Verification items for the finished model (mm, model axes). Coordinates: 2 decimals unless noted, no trailing zeros. Order: outer loops, then holes, each group sorted by start corner. A loop starts at its lowest first (then second) coordinate and runs counter-clockwise, first axis right, second up.
Q1. Cross-section at B-B, the plane x = 5. Record the boundary of the cut face in (y, z).
Q2. Cross-section at C-C, the plane y = 0.75. Record the boundary of the cut face in (x, z).
Q3. Thickness scan on line 1 (X direction, y = 2.65, z = 3); line 2 (Z direction, x = 17, y = 1.95). Record the ranges inside material, lowest first.
Q4. Depth check by flat-ended pin: P1, Ø2.5, axis at x = 17, z = 11, coming from the +Y side. Enter the tip coordinate at first touch or a pass-through.
Q5. Cross-section at A-A, the plane z = 3. Record the boundary of the cut face in (x, y).
Q6. Draft check along Z on faces 1 (the cylindrical face through (15.5, 1.97, 3.07)), 2 (the cylindrical face through (15.5, 1.97, 11.07)), 3 (the flat face through (11, 4, 7)), 4 (the flat face through (11, 2, 0)). Enter one of: pulls with the +Z half, pulls with the -Z half, needs draft (parallel to the pull), parting line crosses it, or undercut.
Autodesk Fusion 360 part; units mm, degrees
sketch "Sketch1" plane through (0, 0, 0) normal (0, 1, 0) x (1, 0, 0)
  line L0 (0, 0) -> (22, 0)
  line L1 (22, 0) -> (22, -15)
  line L2 (22, -15) -> (0, -15)
  line L3 (0, -15) -> (0, 0)
  circle A0 centre (17, -11) radius 1.5
  line L4 (0, -15) -> (0, -14.748)
  circle A1 centre (5, -3) radius 1.5
  circle A2 centre (17, -3) radius 1.5
  circle A3 centre (5, -11) radius 1.5
  dimension "d11" = 3
  dimension "d18" = 3
  dimension "d21" = 3
  dimension "d24" = 3
extrude "Extrude1" add sketch "Sketch1" along normal blind 4 makes body 1
copy_body "Body->Comp1" bodies 1 removing the originals makes body 2 in component "Component"
component "Component" placed x (1, 0, 0) y (0, 1, 0) z (0, 0, 1) at (0, 0, 0)
Check values:
1. outline: (0, 0) - (4, 0) - (4, 1.5) - (0, 1.5) - close; (0, 4.5) - (4, 4.5) - (4, 9.5) - (0, 9.5) - close; (0, 12.5) - (4, 12.5) - (4, 15) - (0, 15) - close
2. outline: (0, 0) - (22, 0) - (22, 15) - (0, 15) - close; hole circle Ø3 at (5, 3); hole circle Ø3 at (5, 11); hole circle Ø3 at (17, 3); hole circle Ø3 at (17, 11)
3. line 1: x = 0 to 3.5, 6.5 to 15.5, 18.5 to 22
3. line 2: z = 0 to 1.5, 4.5 to 9.5, 12.5 to 15
4. P1: passes through
5. outline: (0, 0) - (3.5, 0) - (3.5, 4) - (0, 4) - close; (6.5, 0) - (15.5, 0) - (15.5, 4) - (6.5, 4) - close; (18.5, 0) - (22, 0) - (22, 4) - (18.5, 4) - close
6. face 1: undercut
6. face 2: undercut
6. face 3: needs draft
6. face 4: pulls with the -Z half
